Source: three-view drawing plus pictorial views. Frame: mm from the lowest corner of the part. A direction names the side the tool comes from. Coordinates: 2 decimals unless noted, no trailing zeros. Order: outer loops, then holes, each group sorted by start corner. A loop starts at its lowest first (then second) coordinate and runs counter-clockwise, first axis right, second up. Notation, with made-up numbers: (33.25, 76) -> (78.25, 76) arc R22 cw to (78.25, 103) -> close; hole circle Ø11 at (0, 42). An arc over 180 degrees is marked (long way). One line per question, with ' | ' between items.
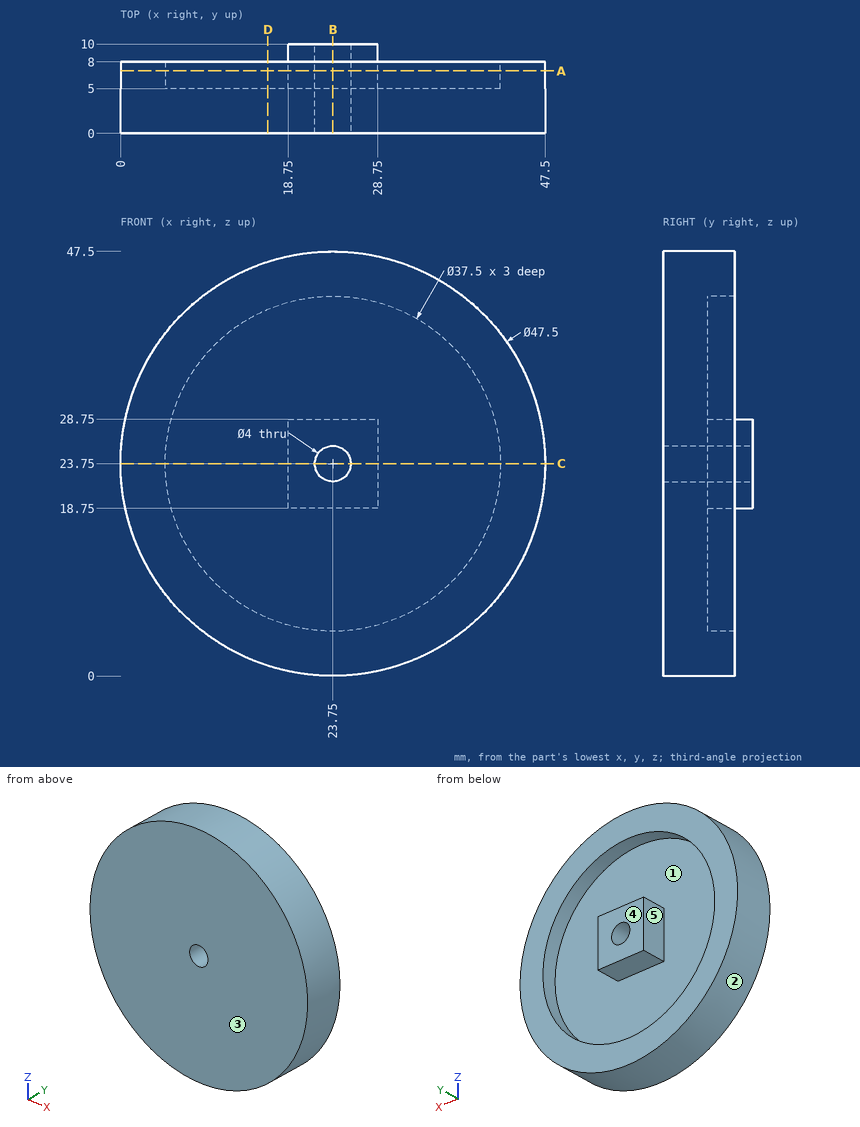
1. Pin query (flat end, axial travel): pin 1 Ø6 at (y, z) = (8.5, 8) entering from +X; pin 2 Ø5.5 at (x, y) = (25.5, 8.5) entering from +Z; pin 3 Ø2 at (y, z) = (5.5, 31) entering from +X. Return the tip coordinate at first contact, or that it passes through.
Recorded:
pin 1: stops at x = 43.76 | pin 2: stops at z = 47.5 | pin 3: stops at x = 46.66
2. Cut plane B-B, the plane x = 23.75. Return loops of the section in (y, z).
Recorded:
outline: (0, 0) -> (8, 0) -> (8, 5) -> (5, 5) -> (5, 18.75) -> (10, 18.75) -> (10, 21.75) -> (0, 21.75) -> close; (0, 25.75) -> (10, 25.75) -> (10, 28.75) -> (5, 28.75) -> (5, 42.5) -> (8, 42.5) -> (8, 47.5) -> (0, 47.5) -> close
3. Cut plane C-C, the plane z = 23.75. Return loops of the section in (x, y).
Recorded:
outline: (0, 0) -> (21.75, 0) -> (21.75, 10) -> (18.75, 10) -> (18.75, 5) -> (5, 5) -> (5, 8) -> (0, 8) -> close; (25.75, 0) -> (47.5, 0) -> (47.5, 8) -> (42.5, 8) -> (42.5, 5) -> (28.75, 5) -> (28.75, 10) -> (25.75, 10) -> close
4. Ray query, line 1 (Z direction, x = 23.75, y = 5.5); line 2 (Z direction, x = 23.75, y = 3.5). Return the intervals inside material, ascending. Write a range as [from, to].
Recorded:
line 1: z = [0, 5], [18.75, 21.75], [25.75, 28.75], [42.5, 47.5] | line 2: z = [0, 21.75], [25.75, 47.5]
5. Mould query, pull axis Z, two halves, no side actions, for the marked faces 1, 2 and 3. Classes: released by +Z, released by -Z, zero draft, split by the parting line, or undercut.
Recorded:
face 1: undercut | face 2: split by the parting line | face 3: zero draft
6. Cut plane A-A, the plane y = 7. Return loops of the section in (x, z).
Recorded:
outline: circle Ø47.5 at (23.75, 23.75); (18.75, 18.75) -> (28.75, 18.75) -> (28.75, 28.75) -> (18.75, 28.75) -> close; hole circle Ø37.5 at (23.75, 23.75); hole circle Ø4 at (23.75, 23.75)
7. Access query for the marked faces 4 and 5. Directions: +Z, -Z, +X, -X, +Y, -Y. A direction counts if a zero-diameter tool reaches every point of the face in a straight line with its end or side. Return the directions, or none.
Recorded:
face 4: +Z, -Z, +X, -X, +Y | face 5: +Y
8. Cut plane D-D, the plane x = 16.5. Return loops of the section in (y, z), and give its area (3 significant figures).
Recorded:
outline: (0, 1.13) -> (8, 1.13) -> (8, 6.46) -> (5, 6.46) -> (5, 41.04) -> (8, 41.04) -> (8, 46.37) -> (0, 46.37) -> close | area: 258 mm^2
